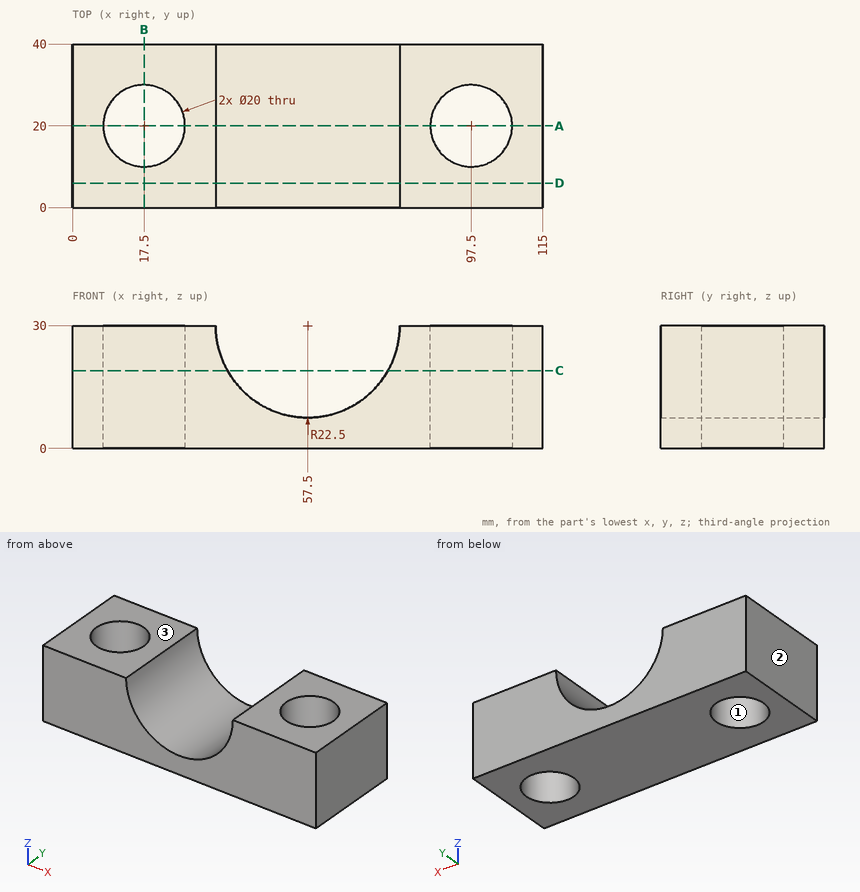
Print and shaded views of the part. All mm, measured from the part's lowest x, y and z. Coordinates: 2 decimals unless noted, no trailing zeros. Order: outer loops, then holes, each group sorted by start corner. A loop starts at its lowest first (then second) coordinate and runs counter-clockwise, first axis right, second up.
(1) Slice it at B-B, the plane x = 17.5. Write the cut outline in (y, z).
Check sheet entries:
outline: (0, 0) - (10, 0) - (10, 30) - (0, 30) - close; (30, 0) - (40, 0) - (40, 30) - (30, 30) - close
(2) Slice it at D-D, the plane y = 6. Write the cut outline in (x, z).
Check sheet entries:
outline: (0, 0) - (115, 0) - (115, 30) - (80, 30) arc R22.5 cw to (35, 30) - (0, 30) - close
(3) Slice it at A-A, the plane y = 20. Write the cut outline in (x, z), and give its area (3 significant figures).
Check sheet entries:
outline: (0, 0) - (7.5, 0) - (7.5, 30) - (0, 30) - close; (27.5, 0) - (87.5, 0) - (87.5, 30) - (80, 30) arc R22.5 cw to (35, 30) - (27.5, 30) - close; (107.5, 0) - (115, 0) - (115, 30) - (107.5, 30) - close
area: 1,450 mm2
(4) Pin check, flat tips, straight feed: pin 1 Ø18 at (x, y) = (17.5, 20) entering from -Z; pin 2 Ø5 at (x, y) = (68, 7.5) entering from +Z. Stop position of each tip, or through.
Check sheet entries:
pin 1: passes through
pin 2: stops at z = 11.64
(5) Pull direction X, two halves, no side cores. Call the marked faces 1, 2 and 3: pulls with the +X half, pulls with the -X half, needs draft (parallel to the pull), parting line crosses it, or undercut.
Check sheet entries:
face 1: undercut
face 2: pulls with the -X half
face 3: needs draft
(6) Slice it at C-C, the plane z = 19. Write the cut outline in (x, y).
Check sheet entries:
outline: (0, 0) - (37.87, 0) - (37.87, 40) - (0, 40) - close; (77.13, 0) - (115, 0) - (115, 40) - (77.13, 40) - close; hole circle Ø20 at (17.5, 20); hole circle Ø20 at (97.5, 20)
(7) Probe L1, parallel to Y at x = 17.5, z = 18.75; L2, parallel to X at y = 21.5, z = 16; L3, parallel to Y at x = 89, z = 20.5. List the from-to ranges inside material, lowest first.
Check sheet entries:
L1: y = 0 to 10, 30 to 40
L2: x = 0 to 7.61, 27.39 to 39.89, 75.11 to 87.61, 107.39 to 115
L3: y = 0 to 14.73, 25.27 to 40
